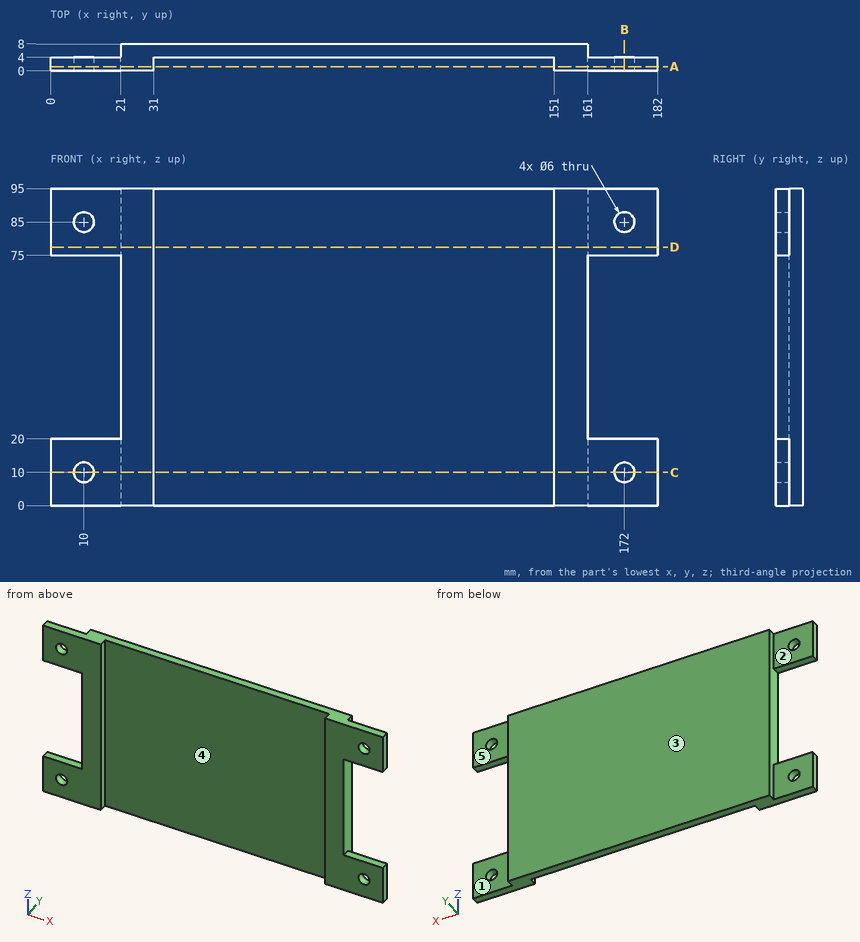
Check sheet for the drawn part. Datum: minimum x, y, z corner. Units: mm. A direction names the side the tool comes from. Coordinates: 2 decimals unless noted, no trailing zeros. Write each loop counter-clockwise with the first axis right and the second up, starting at its lowest first coordinate (ties: lowest second). Pieces come first, ordered by that corner, then holes. Notation, with made-up numbers: (86, -29.5) - (145, -29.5) arc R19 ccw to (145, -22.5) - close; hole circle Ø7 at (66, 83.25). An arc over 180 degrees is marked (long way). Answer as a JSON object with one key per item and string values.
(1) Cross-section at C-C on z = 10. Record the cut outline in (x, y), plus the area to 3 significant figures.
Report:
{"outline": "(0, 0) - (7, 0) - (7, 4) - (0, 4) - close; (13, 0) - (31, 0) - (31, 4) - (151, 4) - (151, 0) - (169, 0) - (169, 4) - (161, 4) - (161, 8) - (21, 8) - (21, 4) - (13, 4) - close; (175, 0) - (182, 0) - (182, 4) - (175, 4) - close", "area": "760 mm^2"}
(2) Mould release check, pull along X, two halves, no side actions. Record for the marked faces 4 and 5: pulls with the +X half, pulls with the -X half, needs draft (parallel to the pull), parting line crosses it, or undercut.
Report:
{"face 4": "undercut", "face 5": "needs draft"}
(3) Tool access check on the marked faces 1, 2 and 3. Record the directions out of +Z, -Z, +X, -X, +Y, -Y that give a thin tool (end or side, any length) a straight path to the whole face; none if there is none.
Report:
{"face 1": "+Z, -Z, +X, +Y", "face 2": "+Z, -Z, -X, +Y", "face 3": "+Z, -Z, +X, -X, +Y"}
(4) Cross-section at B-B on x = 172. Record the cut outline in (y, z), plus the area to 3 significant figures.
Report:
{"outline": "(0, 0) - (4, 0) - (4, 7) - (0, 7) - close; (0, 13) - (4, 13) - (4, 20) - (0, 20) - close; (0, 75) - (4, 75) - (4, 82) - (0, 82) - close; (0, 88) - (4, 88) - (4, 95) - (0, 95) - close", "area": "112 mm^2"}
(5) Thickness scan on line 1 along X through (y, z) = (0.8, 10); line 2 along Z through (x, y) = (10, 3.1); line 3 along X through (y, z) = (2, 21.5). Record the ranges inside material, lowest first.
Report:
{"line 1": "0 to 7, 13 to 31, 151 to 169, 175 to 182", "line 2": "0 to 7, 13 to 20, 75 to 82, 88 to 95", "line 3": "21 to 31, 151 to 161"}
(6) Cross-section at D-D on z = 77.5. Record the cut outline in (x, y).
Report:
{"outline": "(0, 0) - (31, 0) - (31, 4) - (151, 4) - (151, 0) - (182, 0) - (182, 4) - (161, 4) - (161, 8) - (21, 8) - (21, 4) - (0, 4) - close"}
(7) Cross-section at A-A on y = 1.25. Record the cut outline in (x, z), plus the area to 3 significant figures.
Report:
{"outline": "(0, 0) - (31, 0) - (31, 95) - (0, 95) - (0, 75) - (21, 75) - (21, 20) - (0, 20) - close; (151, 0) - (182, 0) - (182, 20) - (161, 20) - (161, 75) - (182, 75) - (182, 95) - (151, 95) - close; hole circle Ø6 at (10, 10); hole circle Ø6 at (10, 85); hole circle Ø6 at (172, 10); hole circle Ø6 at (172, 85)", "area": "3,470 mm^2"}
(8) Gauge pin test, flat ends, axial feed: pin 1 Ø22 at (x, z) = (8, 12) entering from +Y; pin 2 Ø3 at (x, y) = (7, 2.5) entering from -Z; pin 3 Ø8 at (x, z) = (116, 67) entering from -Y; pin 4 Ø5.5 at (x, z) = (10, 85) entering from -Y. Record the tip position at first contact, or that the pin passes through.
Report:
{"pin 1": "y = 4", "pin 2": "z = 0", "pin 3": "y = 4", "pin 4": "through"}
